Could you check a few things on this drawing? It's one solid part, dimensions in mm from its lowest x, y, z. A direction names the side the tool comes from. Give positions to 0.01 mm unless a question says otherwise; leave off trailing zeros. Write each loop counter-clockwise with the first axis right and the second up, starting at its lowest first coordinate (ties: lowest second). Pieces come first, ordered by that corner, then holes. Notation, with made-up numbers: M -24,-17 L 8,-17 A30 ccw 8,7 Z; hole C 45,6 d9. An arc over 180 degrees is marked long. Write each question's results on one line, items separated by ' | '.
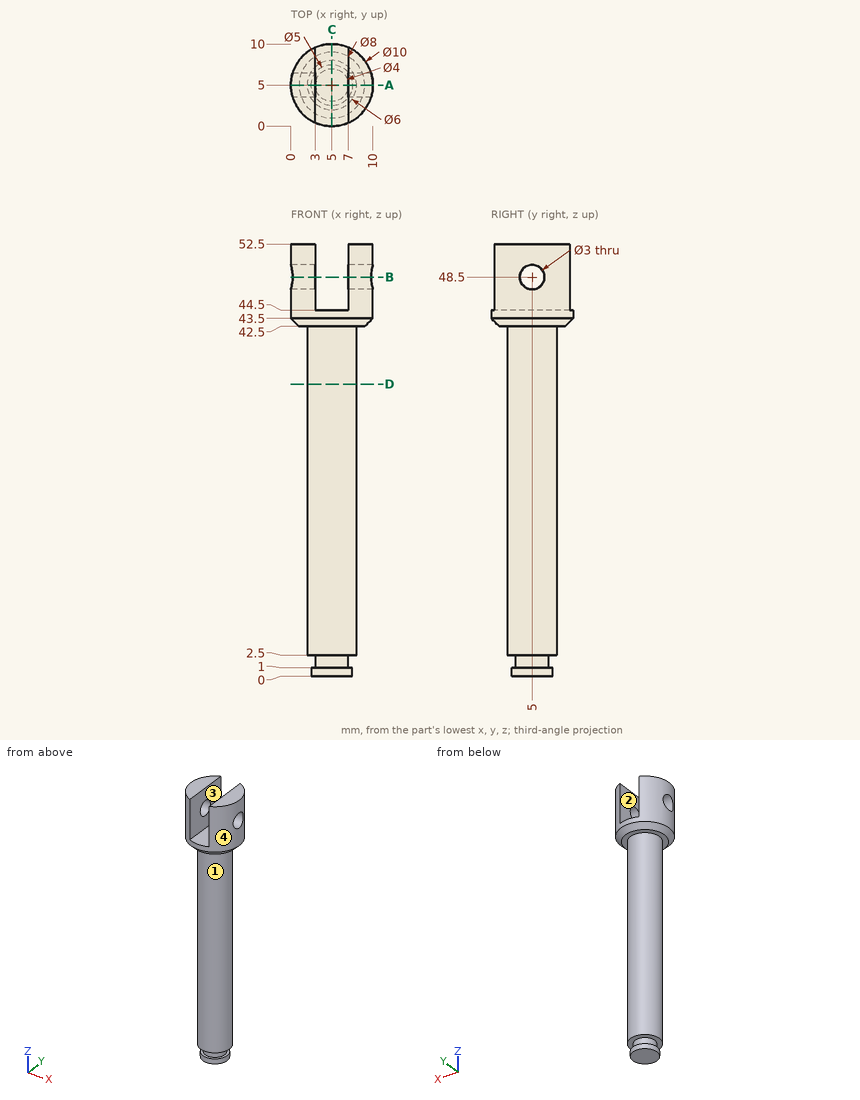
Item 1: If I drill on line 1 (Y direction, x = 8, z = 48.5); line 2 (Z direction, x = 3.25, y = 8.25); line 3 (X direction, y = 7, z = 48.5), over which ranges is the centre line in solid material (lowest first)? Write a range as from..to.
Geometry says:
line 1: y = 1..3.5, 6.5..9 | line 2: z = 42.5..44.5 | line 3: x = 0.42..3, 7..9.58
Item 2: Thinking about a two-plate mould opening in X: for the marked faces 1 and 2, which applies, +X half, -X half, draft (parallel to the pull), parting line (faces both ways), or undercut?
Geometry says:
face 1: parting line | face 2: undercut
Item 3: I'm going to push flat-ended pins straight in: pin 1 (4 mm diameter, centred on y = 5.5, z = 50, fed in from +X); pin 2 (2.5 mm diameter, centred on x = 4.5, y = 5, fed in from +Z); pin 3 (2 mm diameter, centred on x = 1.5, y = 2.5, fed in from -Z); pin 4 (1.5 mm diameter, centred on x = 4, z = 15, fed in from +Y). Where does each tip first touch, or does it pass through?
Geometry says:
pin 1: stops at x = 10 | pin 2: stops at z = 44.5 | pin 3: stops at z = 42.5 | pin 4: stops at y = 7.99
Item 4: I want a section at B-B, the plane z = 48.5. Please give me the cut outline in (x, y).
Geometry says:
outline: M 0.23,3.5 A5 ccw 3,0.42 L 3,3.5 Z; M 0.23,6.5 L 3,6.5 L 3,9.58 A5 ccw Z; M 7,0.42 A5 ccw 9.77,3.5 L 7,3.5 Z; M 7,6.5 L 9.77,6.5 A5 ccw 7,9.58 Z
Item 5: I want a section at C-C, the plane x = 5. Please give me the cut outline in (y, z), and give its area (3 significant figures).
Geometry says:
outline: M 0,43.5 L 1,42.5 L 2,42.5 L 2,2.5 L 3,2.5 L 3,1 L 2.5,1 L 2.5,0 L 7.5,0 L 7.5,1 L 7,1 L 7,2.5 L 8,2.5 L 8,42.5 L 9,42.5 L 10,43.5 L 10,44.5 L 0,44.5 Z | area: 270 mm2
Item 6: I want a section at D-D, the plane z = 35.5. Please give me the cut outline in (x, y).
Geometry says:
outline: C 5,5 d6
Item 7: For the marked faces 3 and 4, which set-ups out of +Z, -Z, +X, -X, +Y, -Y let a thin tool reach every point of the face, with its end or its side?
Geometry says:
face 3: +Z, +Y, -Y | face 4: +Z, -Z
Item 8: I want a section at A-A, the plane y = 5. Give the number of separate pieces and of enclosed holes in the cut face, and give its area (3 significant figures).
Geometry says:
separate pieces: 3 | enclosed holes: 0 | area: 300 mm2
